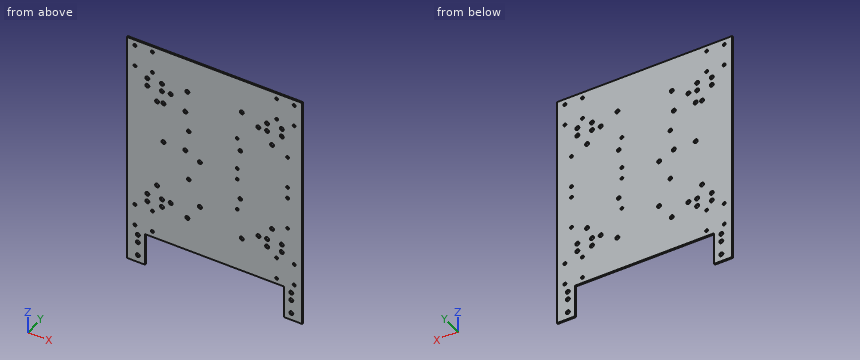
```python
from build123d import *

# Parameters (mm, degrees)
SM_BASE_FLANGE_2_DEPTH   = 2
SKETCH_26_R              = 2
CUT_EXTRUDE_1_DEPTH      = 221.519840377
SKETCH_27_R              = 2.5
CUT_EXTRUDE_2_DEPTH      = 10
SKETCH_28_R              = 2.75
CUT_EXTRUDE_3_DEPTH      = 10
SKETCH_29_R              = 2.75
CUT_EXTRUDE_4_DEPTH      = 10
SKETCH_30_R              = 2.75
CUT_EXTRUDE_5_DEPTH      = 10
MIRROR_3_COPY_1_SKETCH_R = 2.75
MIRROR_3_COPY_1_DEPTH    = 10
SKETCH_31_R              = 2
CUT_EXTRUDE_6_DEPTH      = 10
PATTERN_LINEAR_1_COUNT   = 2
PATTERN_LINEAR_1_PITCH   = 60
SKETCH_32_R              = 2.75
CUT_EXTRUDE_7_DEPTH      = 10
SKETCH_33_R              = 2.75
CUT_EXTRUDE_8_DEPTH      = 10


# Sheet-metal steps are written as plain solids
with BuildPart() as part:
    # 草图2 → 基体-法兰2 (new body)
    with BuildSketch(Plane(origin=(0, 0, 0), x_dir=(1, 0, 0), z_dir=(0, 1, 0))):
        Polygon((-120, 140), (-120, 185), (-95, 185), (-95, 140), (95, 140), (95, 185), (120, 185), (120, 140), (120, -140), (-120, -140), align=None)
    extrude(amount=-SM_BASE_FLANGE_2_DEPTH)

    # 草图26 → 切除-拉伸1 (cut, through all)
    with BuildSketch(Plane(origin=(0, 0, 0), x_dir=(1, 0, 0), z_dir=(0, 1, 0))):
        with Locations(Location((-109, 102, 0), (0, 0, 270))):
            Circle(SKETCH_26_R)
        with Locations(Location((-109, 132, 0), (0, 0, 270))):
            Circle(SKETCH_26_R)
        with Locations(Location((-85, 132, 0), (0, 0, 270))):
            Circle(SKETCH_26_R)
        with Locations(Location((-85, 102, 0), (0, 0, 270))):
            Circle(SKETCH_26_R)
        with Locations(Location((-85, -102, 0), (0, 0, 90))):
            Circle(SKETCH_26_R)
        with Locations(Location((-85, -132, 0), (0, 0, 90))):
            Circle(SKETCH_26_R)
        with Locations(Location((-109, -132, 0), (0, 0, 90))):
            Circle(SKETCH_26_R)
        with Locations(Location((-109, -102, 0), (0, 0, 90))):
            Circle(SKETCH_26_R)
        with Locations(Location((85, 102, 0), (0, 0, 90))):
            Circle(SKETCH_26_R)
        with Locations(Location((85, 132, 0), (0, 0, 90))):
            Circle(SKETCH_26_R)
        with Locations(Location((109, 132, 0), (0, 0, 90))):
            Circle(SKETCH_26_R)
        with Locations(Location((109, 102, 0), (0, 0, 90))):
            Circle(SKETCH_26_R)
        with Locations(Location((109, -102, 0), (0, 0, 270))):
            Circle(SKETCH_26_R)
        with Locations(Location((109, -132, 0), (0, 0, 270))):
            Circle(SKETCH_26_R)
        with Locations(Location((85, -132, 0), (0, 0, 270))):
            Circle(SKETCH_26_R)
        with Locations(Location((85, -102, 0), (0, 0, 270))):
            Circle(SKETCH_26_R)
    extrude(amount=-CUT_EXTRUDE_1_DEPTH, mode=Mode.SUBTRACT)

    # 草图27 → 切除-拉伸2 (cut)
    with BuildSketch(Plane.XZ.offset(2)):
        with Locations(Location((-35.355339059, 35.355339059, 0), (0, 0, 270))):
            Circle(SKETCH_27_R)
        with Locations(Location((35.355339059, 35.355339059, 0), (0, 0, 270))):
            Circle(SKETCH_27_R)
        with Locations(Location((35.355339059, -35.355339059, 0), (0, 0, 270))):
            Circle(SKETCH_27_R)
        with Locations(Location((-35.355339059, -35.355339059, 0), (0, 0, 270))):
            Circle(SKETCH_27_R)
    extrude(amount=-CUT_EXTRUDE_2_DEPTH, mode=Mode.SUBTRACT)

    # 草图28 → 切除-拉伸3 (cut)
    with BuildSketch(Plane.XZ.offset(2)):
        with Locations(Location((-60, -80, 0), (0, 0, 270))):
            Circle(SKETCH_28_R)
        with Locations(Location((-37.250025969, -92.803208809, 0), (0, 0, 270))):
            Circle(SKETCH_28_R)
        with Locations(Location((-78.661073186, -61.744923397, 0), (0, 0, 270))):
            Circle(SKETCH_28_R)
        with Locations(Location((78.661073186, -61.744923397, 0), (0, 0, 90))):
            Circle(SKETCH_28_R)
        with Locations(Location((37.250025969, -92.803208809, 0), (0, 0, 90))):
            Circle(SKETCH_28_R)
        with Locations(Location((60, -80, 0), (0, 0, 90))):
            Circle(SKETCH_28_R)
        with Locations(Location((-78.661073186, 61.744923397, 0), (0, 0, 90))):
            Circle(SKETCH_28_R)
        with Locations(Location((-37.250025969, 92.803208809, 0), (0, 0, 90))):
            Circle(SKETCH_28_R)
        with Locations(Location((-60, 80, 0), (0, 0, 90))):
            Circle(SKETCH_28_R)
        with Locations(Location((60, 80, 0), (0, 0, 270))):
            Circle(SKETCH_28_R)
        with Locations(Location((37.250025969, 92.803208809, 0), (0, 0, 270))):
            Circle(SKETCH_28_R)
        with Locations(Location((78.661073186, 61.744923397, 0), (0, 0, 270))):
            Circle(SKETCH_28_R)
    extrude(amount=-CUT_EXTRUDE_3_DEPTH, mode=Mode.SUBTRACT)

    # 草图29 → 切除-拉伸4 (cut)
    with BuildSketch(Plane.XZ.offset(2)):
        with Locations(Location((105, -175, 0), (0, 0, 270))):
            Circle(SKETCH_29_R)
        with Locations(Location((105, -156, 0), (0, 0, 270))):
            Circle(SKETCH_29_R)
        with Locations(Location((105, -145, 0), (0, 0, 270))):
            Circle(SKETCH_29_R)
    cut_extrude_4 = extrude(amount=-CUT_EXTRUDE_4_DEPTH, mode=Mode.SUBTRACT)

    # 镜向1: 切除-拉伸4 across plane
    add(cut_extrude_4.mirror(Plane(origin=(0, 0, 0), x_dir=(0, 0, 1), z_dir=(1, 0, 0))), mode=Mode.SUBTRACT)

    # 草图30 → 切除-拉伸5 (cut)
    with BuildSketch(Plane(origin=(0, 0, 0), x_dir=(1, 0, 0), z_dir=(0, 1, 0))):
        with Locations(Location((-92, 90.5, 0), (0, 0, 270))):
            Circle(SKETCH_30_R)
        with Locations(Location((-92, 79.5, 0), (0, 0, 270))):
            Circle(SKETCH_30_R)
        with Locations(Location((-72, 79.5, 0), (0, 0, 270))):
            Circle(SKETCH_30_R)
        with Locations(Location((-72, 90.5, 0), (0, 0, 270))):
            Circle(SKETCH_30_R)
    cut_extrude_5 = extrude(amount=-CUT_EXTRUDE_5_DEPTH, mode=Mode.SUBTRACT)

    # 镜向2: 切除-拉伸5 across plane
    add(cut_extrude_5.mirror(Plane.XY), mode=Mode.SUBTRACT)

    # 镜向3: 切除-拉伸5 across plane
    add(cut_extrude_5.mirror(Plane(origin=(0, 0, 0), x_dir=(0, 0, 1), z_dir=(1, 0, 0))), mode=Mode.SUBTRACT)

    # 镜向3 copy 1 sketch → 镜向3 copy 1 (cut)
    with BuildSketch(Plane(origin=(0, 0, 0), x_dir=(-1, 0, 0), z_dir=(0, 1, 0))):
        with Locations(Location((-92, 90.5, 0), (0, 0, 270))):
            Circle(MIRROR_3_COPY_1_SKETCH_R)
        with Locations(Location((-92, 79.5, 0), (0, 0, 270))):
            Circle(MIRROR_3_COPY_1_SKETCH_R)
        with Locations(Location((-72, 79.5, 0), (0, 0, 270))):
            Circle(MIRROR_3_COPY_1_SKETCH_R)
        with Locations(Location((-72, 90.5, 0), (0, 0, 270))):
            Circle(MIRROR_3_COPY_1_SKETCH_R)
    extrude(amount=-MIRROR_3_COPY_1_DEPTH, mode=Mode.SUBTRACT)

    # 草图31 → 切除-拉伸6 (cut)
    with BuildSketch(Plane(origin=(0, 0, 0), x_dir=(1, 0, 0), z_dir=(0, 1, 0))):
        with Locations(Location((31.05, -52, 0), (0, 0, 270))):
            Circle(SKETCH_31_R)
        with Locations(Location((31.05, -7.74, 0), (0, 0, 270))):
            Circle(SKETCH_31_R)
        with Locations(Location((100, -7.74, 0), (0, 0, 270))):
            Circle(SKETCH_31_R)
        with Locations(Location((100, -52, 0), (0, 0, 270))):
            Circle(SKETCH_31_R)
    cut_extrude_6 = extrude(amount=-CUT_EXTRUDE_6_DEPTH, mode=Mode.SUBTRACT)

    # 阵列(线性)1: 切除-拉伸6 ×2
    with Locations(*[(0, 0, -i * PATTERN_LINEAR_1_PITCH) for i in range(1, PATTERN_LINEAR_1_COUNT)]):
        add(cut_extrude_6, mode=Mode.SUBTRACT)

    # 草图32 → 切除-拉伸7 (cut)
    with BuildSketch(Plane(origin=(0, 0, 0), x_dir=(1, 0, 0), z_dir=(0, 1, 0))):
        with Locations(Location((-20, 69.5, 0), (0, 0, 270))):
            Circle(SKETCH_32_R)
        with Locations(Location((-20, 3.8, 0), (0, 0, 270))):
            Circle(SKETCH_32_R)
    extrude(amount=-CUT_EXTRUDE_7_DEPTH, mode=Mode.SUBTRACT)

    # 草图33 → 切除-拉伸8 (cut)
    with BuildSketch(Plane(origin=(0, 0, 0), x_dir=(1, 0, 0), z_dir=(0, 1, 0))):
        with Locations(Location((-70, -62.5, 0), (0, 0, 270))):
            Circle(SKETCH_33_R)
        with Locations(Location((-70, -5.5, 0), (0, 0, 270))):
            Circle(SKETCH_33_R)
        with Locations(Location((-40, -5.5, 0), (0, 0, 270))):
            Circle(SKETCH_33_R)
        with Locations(Location((-40, -62.5, 0), (0, 0, 270))):
            Circle(SKETCH_33_R)
    extrude(amount=-CUT_EXTRUDE_8_DEPTH, mode=Mode.SUBTRACT)


solid = part.part
```
Source: CAD feature listing. Evaluate the final solid. Frame: model axes, mm. Coordinates: 2 decimals unless noted, no trailing zeros. Loops run counter-clockwise (first coordinate to the right, second up) from the corner with the lowest first, then second, coordinate; pieces in that order, holes last. Notation, with made-up numbers: (32, 55) - (60, 55) arc R14 ccw to (60, 63) - close; hole circle Ø9 at (70.25, 48.5). An arc over 180 degrees is marked (long way). Answer as CSV lines item,"result".
1. Section A-A (x = -12). Return loops of the section in (y, z), then the cut area to 3 significant figures.
Established:
outline,"(-2, -140) - (0, -140) - (0, 140) - (-2, 140) - close"
area,"560 mm2"
2. Ray query, line 1 (X direction, y = -0.45, z = 132); line 2 (X direction, y = -0.8, z = 35.5); line 3 (Z direction, x = 108.5, y = -1.2). Return the intervals inside material, ascending.
Established:
line 1,"x = -120 to -111, -107 to -87, -83 to 83, 87 to 107, 111 to 120"
line 2,"x = -120 to -37.85, -32.86 to 32.86, 37.85 to 120"
line 3,"z = -185 to -133.94, -130.06 to -103.94, -100.06 to 100.06, 103.94 to 130.06, 133.94 to 140"
3. Section B-B (y = -0.35). Count the separate pieces of the cut face and the enclosed holes in it, then the cut area to 3 significant figures.
Established:
separate pieces,"1"
enclosed holes,"68"
area,"68,100 mm2"
